Geometry: see drawing. Coordinates: mm, zero at the bounding-box minimum. A direction names the side the tool comes from. Coordinates: 2 decimals unless noted, no trailing zeros. Write each loop counter-clockwise with the first axis right and the second up, starting at its lowest first coordinate (ties: lowest second). Pieces come first, ordered by that corner, then holes. Notation, with made-up numbers: M 28,83.5 L 48,83.5 A19 ccw 48,97.5 Z; hole C -30.75,-31 d6. An arc over 180 degrees is marked long. Answer as CSV lines item,"result". Start each with the question number.
1. Line query: probe 1 along Z at (x, y) = (63.5, 27.5); probe 2 along X at (y, z) = (14, 2.5); probe 3 along X at (y, z) = (19.05, 5.5) (1 decimal). Output: solid intervals per line, ascending. Write a range as [from, to].
2. Section B-B on z = 9. Return the cut outline in (x, y), plus the area to 3 significant figures.
3. Section D-D on z = 17. Return the cut outline in (x, y) (1 decimal), plus the area to 3 significant figures.
4. Contact query for a flat-ended pin moving along its axis: pin 1 Ø16.5 at (x, y) = (109, 10.5) entering from +Z. Output: stop coordinate, or through.
5. Reachability of the marked faces 1 and 2 from +Z, -Z, +X, -X, +Y, -Y: full face, straight path, thin tool, end or side. Return the list, or none.
6. Section A-A on y = 21.5. Return the cut outline in (x, z) (1 decimal), plus the area to 3 significant figures.
7. Section C-C on x = 19.05. Return the cut outline in (y, z).
8. Mould query, pull axis X, two halves, no side actions, for the marked faces 3, 4 and 5. Classes: pulls with the +X half, pulls with the -X half, needs draft (parallel to the pull), parting line crosses it, or undercut.
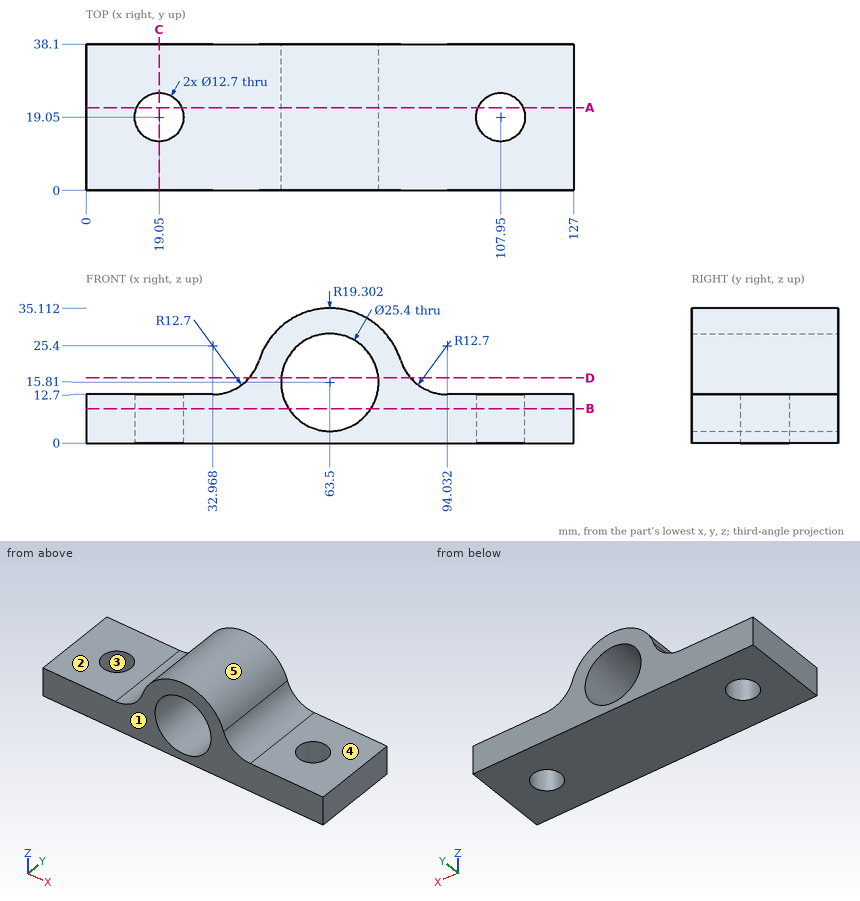
Values:
1,probe 1,"[0, 3.11], [28.51, 35.11]"
1,probe 2,"[0, 15.2], [22.9, 104.1], [111.8, 127]"
1,probe 3,"[0, 12.7], [25.4, 56.1], [70.9, 101.6], [114.3, 127]"
2,outline,"M 0,0 L 52.78,0 L 52.78,38.1 L 0,38.1 Z; M 74.22,0 L 127,0 L 127,38.1 L 74.22,38.1 Z; hole C 19.05,19.05 d12.7; hole C 107.95,19.05 d12.7"
2,area,"3,770 mm²"
3,outline,"M 42.5,0 L 50.9,0 L 50.9,38.1 L 42.5,38.1 Z; M 76.1,0 L 84.5,0 L 84.5,38.1 L 76.1,38.1 Z"
3,area,"637 mm²"
4,pin 1,"z = 12.7"
5,face 1,"+Z, -Z, +X, -X, -Y"
5,face 2,"+Z, -X, +Y, -Y"
6,outline,"M 0,0 L 13.2,0 L 13.2,12.7 L 0,12.7 Z; M 24.9,0 L 102.1,0 L 102.1,12.7 L 94,12.7 A12.7 cw 81.9,21.6 A19.3 ccw 45.1,21.6 A12.7 cw 33,12.7 L 24.9,12.7 Z; M 113.8,0 L 127,0 L 127,12.7 L 113.8,12.7 Z; hole C 63.5,15.8 d25.4"
6,area,"1,560 mm²"
7,outline,"M 0,0 L 12.7,0 L 12.7,12.7 L 0,12.7 Z; M 25.4,0 L 38.1,0 L 38.1,12.7 L 25.4,12.7 Z"
8,face 3,"undercut"
8,face 4,"needs draft"
8,face 5,"parting line crosses it"
